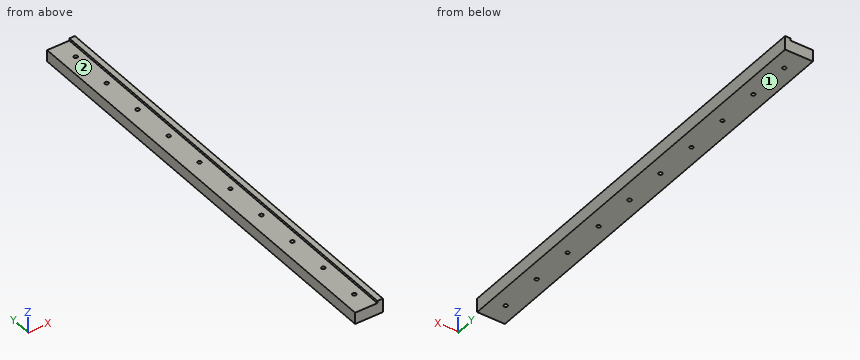
from build123d import *

# Parameters (mm, degrees)
F0_W     = 38.1
F0_H     = 19.05
F1_DEPTH = 596.9
F2_W     = 30.55
F2_H     = 3.175
F3_DEPTH = 596.901
F5_D     = 5.1054
F5_DEPTH = 16.5100084667
F5_TIP   = 1.5338169022


with BuildPart() as f1:
    # F0 (on Front) → F1 (new body)
    with BuildSketch(Plane.XZ):
        Rectangle(F0_W, F0_H)
    extrude(amount=F1_DEPTH)

    # F2 (on face) → F3 (cut, through all)
    with BuildSketch(Plane.XZ.offset(596.9)):
        with Locations((-3.775, 7.9375)):
            Rectangle(F2_W, F2_H)
    extrude(amount=-F3_DEPTH, mode=Mode.SUBTRACT)

    # F5
    with Locations(Plane.XY.offset(6.35)):
        with Locations((0, -568.44946), (0, -508.44946), (0, -448.44946), (0, -388.44946), (0, -328.44946), (0, -268.44946), (0, -208.44946), (0, -148.44946), (0, -88.44946), (0, -28.44946)):
            Hole(F5_D / 2, depth=F5_DEPTH)
            with Locations((0, 0, -(F5_DEPTH + F5_TIP / 2))):  # 118° drill point
                Cone(0, F5_D / 2, F5_TIP, mode=Mode.SUBTRACT)


solid = f1.part
Build history of the part. All positions in model axes, mm. Face numbers are marked on the shaded views. A direction names the side the tool comes from. Coordinates: 2 decimals unless noted, no trailing zeros. Write each loop counter-clockwise with the first axis right and the second up, starting at its lowest first coordinate (ties: lowest second). Pieces come first, ordered by that corner, then holes.
(1) Cut at B-B on x = -14. List the corners of the cut face in (y, z) (3 decimals).
(2) Drill centre lines: line 1 (Z direction, x = 7.5, y = -212) (3 decimals); line 2 (X direction, y = -329, z = 7.75). Where is each one in solid material? Low to high.
(3) 3-axis set-ups, long thin cutter, end or side, ignore diameter. For the marked faces 1 and 2: which of +Z, -Z, +X, -X, +Y, -Y reach the whole face in a straight line?
(4) Pin check, flat tips, straight feed: pin 1 Ø8 at (x, y) = (0, -28.45) entering from +Z; pin 2 Ø2 at (x, z) = (-11, 2.5) entering from +Y; pin 3 Ø1.6 at (y, z) = (-367.5, 8) entering from -X. Stop position of each tip, or through.
(5) Cut at A-A on y = -320.5. List the corners of the cut face in (x, z) (3 decimals), and give its area (3 significant figures).
Working result:
1. outline: (-596.9, -9.525) - (0, -9.525) - (0, 6.35) - (-596.9, 6.35) - close
2. line 1: z = -9.525 to 6.35
2. line 2: x = 11.5 to 19.05
3. face 1: -Z, +X, -X, +Y, -Y
3. face 2: +Z, -X, +Y, -Y
4. pin 1: stops at z = 6.35
4. pin 2: stops at y = 0
4. pin 3: stops at x = 11.5
5. outline: (-19.05, -9.525) - (19.05, -9.525) - (19.05, 9.525) - (11.5, 9.525) - (11.5, 6.35) - (-19.05, 6.35) - close
5. area: 629 mm2
